Check sheet for the drawn part. Datum: minimum x, y, z corner. Units: mm. A direction names the side the tool comes from. Round coordinates to 2 decimals unless told otherwise and drop trailing zeros. Write each loop counter-clockwise with the first axis right and the second up, starting at its lowest first coordinate (ties: lowest second). Pieces come first, ordered by that corner, then holes. Notation, with made-up numbers: M 72.5,25 L 84.5,25 A34 cw 84.5,63 Z; hole C -31,57.5 d2. An arc over 180 degrees is marked long. One line per item, written item: value. Start each with the question number.
Item 1: Section check C-C, the plane y = 1.5. Record the cut outline in (x, z) (1 decimal), then the cut area to 3 significant figures.
Item 2: Tool access check on the marked faces 1 and 2. Record the directions out of +Z, -Z, +X, -X, +Y, -Y that give a thin tool (end or side, any length) a straight path to the whole face; none if there is none.
Item 3: Section check D-D, the plane x = 2.5. Record the cut outline in (y, z).
Item 4: Draft check along X on the marked faces 3, 4, 5 and 6. Enter one of: +X half, -X half, draft (parallel to the pull), parting line (faces both ways), or undercut.
Item 5: Section check B-B, the plane z = 4. Record the cut outline in (x, y) (1 decimal).
Item 6: Gauge pin test, flat ends, axial feed: pin 1 (4 mm diameter, centred on y = 4.5, z = 10.5, fed in from -X); pin 2 (4 mm diameter, centred on y = 6, z = 10, fed in from +X); pin 3 (4 mm diameter, centred on y = 2, z = 12.5, fed in from +X). Record the tip position at first contact, or that the pin passes through.
Item 7: Section check A-A, the plane x = 4.5. Record the cut outline in (y, z).
Item 8: Thickness scan on probe 1 along Z at (x, y) = (2.25, 6.25); probe 2 along X at (y, z) = (1.75, 5.5) (1 decimal); probe 3 along X at (y, z) = (6.25, 17.5) (1 decimal). Record the ranges inside material, lowest first. Write a range as from..to.
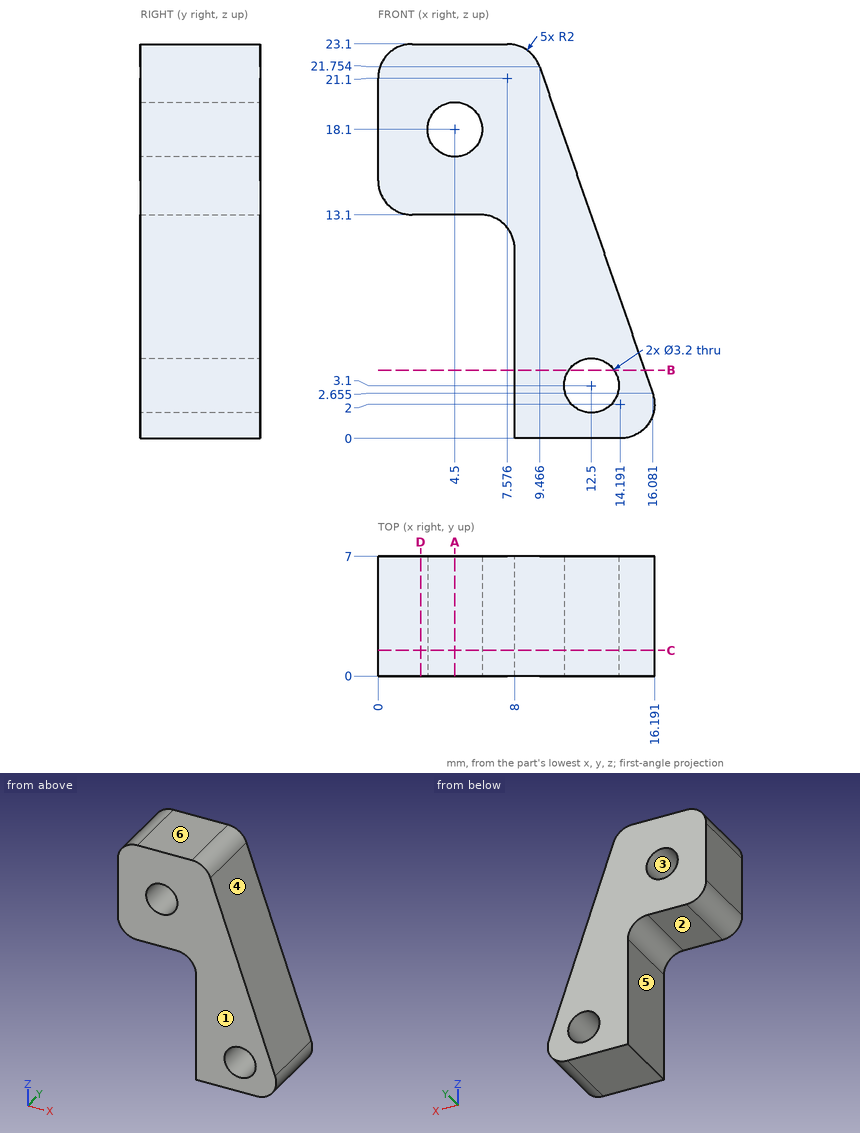
Response values:
1. outline: M 0,15.1 A2 ccw 2,13.1 L 6,13.1 A2 cw 8,11.1 L 8,0 L 14.2,0 A2 ccw 16.1,2.7 L 9.5,21.8 A2 ccw 7.6,23.1 L 2,23.1 A2 ccw 0,21.1 Z; hole C 4.5,18.1 d3.2; hole C 12.5,3.1 d3.2
1. area: 176 mm2
2. face 1: +Z, -Z, +X, -X, -Y
2. face 2: -Z, -X, +Y, -Y
3. outline: M 0,13.1 L 7,13.1 L 7,23.1 L 0,23.1 Z
4. face 3: undercut
4. face 4: +X half
4. face 5: -X half
4. face 6: draft
5. outline: M 8,0 L 11.2,0 L 11.2,7 L 8,7 Z; M 13.8,0 L 15.6,0 L 15.6,7 L 13.8,7 Z
6. pin 1: stops at x = 7.43
6. pin 2: stops at x = 14.23
6. pin 3: stops at x = 13.36
7. outline: M 0,13.1 L 7,13.1 L 7,16.5 L 0,16.5 Z; M 0,19.7 L 7,19.7 L 7,23.1 L 0,23.1 Z
8. probe 1: z = 13.1..23.1
8. probe 2: x = 8..15.1
8. probe 3: x = 0..3, 6..10.9
